Geometry check sheet. Reference: the model listing, model coordinates, mm. Face numbers are marked on the shaded views. A direction names the side the tool comes from. Give positions to 0.01 mm unless a question says otherwise; leave off trailing zeros. Loops run counter-clockwise (first coordinate to the right, second up) from the corner with the lowest first, then second, coordinate; pieces in that order, holes last. Notation, with made-up numbers: (12, 52) -> (71, 52) arc R31 ccw to (71, 76) -> close; hole circle Ø7 at (32, 79). An arc over 180 degrees is marked (long way). One line per item, written item: value. Start each with the question number.
(1) Sectioned sample at B-B, the plane x = -14. Record the cut outline in (y, z) (3 decimals), then the cut area to 3 significant figures.
(2) Scan lines: line 1 along Z through (x, y) = (-53.5, 7) (3 decimals); line 2 along Z through (x, y) = (-17, -2) (3 decimals); line 3 along X through (y, z) = (-17.5, -106). Record each from-to range of solid material in increasing order. Write a range as from..to.
(3) Tool access check on the marked faces 1, 2, 3, 4 and 5. Record the directions out of +Z, -Z, +X, -X, +Y, -Y that give a thin tool (end or side, any length) a straight path to the whole face; none if there is none.
(4) Sectioned sample at C-C, the plane z = -66.5. Record the cut outline in (x, y), then the cut area to 3 significant figures.
(5) Gauge pin test, flat ends, axial feed: pin 1 Ø11.5 at (x, y) = (-24.5, -7.5) entering from -Z; pin 2 Ø10 at (x, z) = (-1.5, -98.5) entering from +Y; pin 3 Ø19 at (y, z) = (8, -49) entering from +X; pin 4 Ø5 at (y, z) = (-9, -111.5) entering from +X. Record the tip position at first contact, or that the pin passes through.
(6) Sectioned sample at D-D, the plane y = -9. State how many separate pieces and enclosed holes the cut face has, then the cut area to 3 significant figures.
(7) Sectioned sample at A-A, the plane x = -39.5. Record the cut outline in (y, z) (3 decimals).
(8) Draft check along X on the marked faces 6, 7, 8 and 9. Enter one of: pulls with the +X half, pulls with the -X half, needs draft (parallel to the pull), parting line crosses it, or undercut.
from build123d import *

# Parameters (mm, degrees)
F1_DEPTH     = 19.05
F6_T1_DEPTH  = 38.1
F6_T3_DEPTH  = 19.05
F6_T5_DEPTH  = 19.05
F6_T10_ANGLE = 45.2137620144
F6_T16_ANGLE = 107.7622686142
F6_T22_ANGLE = 107.7622686142
F6_T25_DEPTH = 69.8548284901
F7_R         = 1.8415
F8_DEPTH     = 38.1010001


# Not quite as in the source:
# - a fillet or chamfer that OpenCascade refuses, or shapes differently, is made with other operations: its cross-section is extruded or revolved along the edge and cut away or added


with BuildPart() as f1:
    # F0 (on Front) → F1 (new body, symmetric)
    with BuildSketch(Plane.XZ):
        Polygon((-63.5, 0), (0, 0), (0, -16.2306), (-63.5, -16.2306), (-63.5, -124.1806), (-25.4, -124.1806), (-25.4, -101.9556), (-31.75, -101.9556), (-31.75, -111.4806), (-50.8, -111.4806), (-50.8, -89.2556), (12.7, -89.2556), (12.7, -70.2056), (6.35, -70.2056), (6.35, -76.5556), (-50.8, -76.5556), (-50.8, -25.7556), (12.7, -25.7556), (12.7, 9.525), (-63.5, 9.525), align=None)
    extrude(amount=F1_DEPTH, both=True)

    # F2 (on Front) → F3 (revolve, cut)
    with BuildSketch(Plane.XZ):
        Polygon((-50.8, -57.5056), (-50.8, -76.5556), (6.35, -76.5556), (6.35, -70.2056), (12.7, -70.2056), (12.7, -57.5056), align=None)
    revolve(axis=Axis((-20.4399991781, 0, -165.4556), (1, 0, 0)), mode=Mode.SUBTRACT)

    # F4 (on Front) → F5 (revolve, cut)
    with BuildSketch(Plane.XZ):
        Polygon((-50.8, -89.2556), (-50.8, -111.4806), (-31.75, -111.4806), (-31.75, -101.9556), (-25.4, -101.9556), (-25.4, -89.2556), align=None)
    revolve(axis=Axis((-41.275, 0, -149.5806), (1, 0, 0)), mode=Mode.SUBTRACT)

    # F6: fillet of radius 6.35 on 13 edges, made by hand

    # F6_s2 → F6_t1 (join)
    with BuildSketch(Plane.XZ.offset(-19.05)):
        with BuildLine():
            ThreePointArc((-44.4490343146, -25.7552), (-48.9401280605, -27.6154719395), (-50.8004, -32.1065656854))
            Line((-50.8004, -32.1065656854), (-51.4355365685, -32.1065656854))
            ThreePointArc((-51.4355365685, -32.1065656854), (-51.4351365685, -28.9310828427), (-51.4351365685, -25.7556))
            Line((-51.4351365685, -25.7556), (-50.8, -25.1204634315))
            ThreePointArc((-50.8, -25.1204634315), (-47.6245171573, -25.1204634315), (-44.4490343146, -25.1200634315))
            Line((-44.4490343146, -25.1200634315), (-44.4490343146, -25.7552))
        make_face()
    extrude(amount=F6_T1_DEPTH)

    # F6_s4 → F6_t3 (join)
    with BuildSketch(Plane.XZ.offset(-19.05)):
        with BuildLine():
            ThreePointArc((-44.4490343146, -89.2552), (-48.9401280605, -91.1154719395), (-50.8004, -95.6065656854))
            Line((-50.8004, -95.6065656854), (-51.4355365685, -95.6065656854))
            ThreePointArc((-51.4355365685, -95.6065656854), (-51.4351365685, -92.4310828427), (-51.4351365685, -89.2556))
            Line((-51.4351365685, -89.2556), (-50.8, -88.6204634315))
            ThreePointArc((-50.8, -88.6204634315), (-47.6245171573, -88.6204634315), (-44.4490343146, -88.6200634315))
            Line((-44.4490343146, -88.6200634315), (-44.4490343146, -89.2552))
        make_face()
    extrude(amount=F6_T3_DEPTH)

    # F6_s6 → F6_t5 (join)
    with BuildSketch(Plane.XZ):
        with BuildLine():
            ThreePointArc((-44.4490343146, -89.2552), (-48.9401280605, -91.1154719395), (-50.8004, -95.6065656854))
            Line((-50.8004, -95.6065656854), (-51.4355365685, -95.6065656854))
            ThreePointArc((-51.4355365685, -95.6065656854), (-51.4351365685, -92.4310828427), (-51.4351365685, -89.2556))
            Line((-51.4351365685, -89.2556), (-50.8, -88.6204634315))
            ThreePointArc((-50.8, -88.6204634315), (-47.6245171573, -88.6204634315), (-44.4490343146, -88.6200634315))
            Line((-44.4490343146, -88.6200634315), (-44.4490343146, -89.2552))
        make_face()
    extrude(amount=F6_T5_DEPTH)


with BuildPart() as f6_tool8:
    # F6_s9 → F6_t10 (revolve)
    with BuildSketch(Plane(origin=(0, -58.7152257849, -24.4490632784), x_dir=(1, 0, 0), z_dir=(0, -0.923164058, -0.384406194))):
        with BuildLine():
            ThreePointArc((-50.8004, -57.4916974353), (-48.9401280605, -61.9827911812), (-44.4490343146, -63.8430631207))
            Line((-44.4490343146, -63.8430631207), (-44.4490343146, -64.4781996892))
            ThreePointArc((-44.4490343146, -64.4781996892), (-47.6245171573, -64.4777996892), (-50.8, -64.4777996892))
            Line((-50.8, -64.4777996892), (-51.4351365685, -63.8426631207))
            ThreePointArc((-51.4351365685, -63.8426631207), (-51.4351365685, -60.667180278), (-51.4355365685, -57.4916974353))
            Line((-51.4355365685, -57.4916974353), (-50.8004, -57.4916974353))
        make_face()
    revolve(axis=Axis((-50.8, 0, -165.4556), (-1, 0, 0)), revolution_arc=F6_T10_ANGLE)

    split(bisect_by=Plane.XZ.offset(19.05), keep=Keep.BOTTOM)

    split(bisect_by=Plane.XZ.offset(-19.05), keep=Keep.TOP)


with BuildPart() as f1_1:
    add(f1.part)

    # F6_t7: union F6_tool8
    add(f6_tool8.part)


with BuildPart() as f6_tool14:
    # F6_s15 → F6_t16 (revolve)
    with BuildSketch(Plane(origin=(0, -71.2250836382, -97.6064441708), x_dir=(1, 0, 0), z_dir=(0, -0.589462371, -0.8077958363))):
        with BuildLine():
            ThreePointArc((-50.8004, -43.7211694448), (-48.9401280605, -48.2122631908), (-44.4490343146, -50.0725351302))
            Line((-44.4490343146, -50.0725351302), (-44.4490343146, -50.7076716988))
            ThreePointArc((-44.4490343146, -50.7076716988), (-47.6245171573, -50.7072716988), (-50.8, -50.7072716988))
            Line((-50.8, -50.7072716988), (-51.4351365685, -50.0721351302))
            ThreePointArc((-51.4351365685, -50.0721351302), (-51.4351365685, -46.8966522875), (-51.4355365685, -43.7211694448))
            Line((-51.4355365685, -43.7211694448), (-50.8004, -43.7211694448))
        make_face()
    revolve(axis=Axis((-50.8, 0, -149.5806), (-1, 0, 0)), revolution_arc=F6_T16_ANGLE)

    split(bisect_by=Plane.XZ.offset(19.05), keep=Keep.BOTTOM)

    split(bisect_by=Plane.XZ.offset(-19.05), keep=Keep.TOP)


with BuildPart() as f1_2:
    add(f1_1.part)

    # F6_t13: union F6_tool14
    add(f6_tool14.part)


with BuildPart() as f6_tool20:
    # F6_s21 → F6_t22 (revolve)
    with BuildSketch(Plane(origin=(0, -71.2250836382, -97.6064441708), x_dir=(1, 0, 0), z_dir=(0, -0.589462371, -0.8077958363))):
        with BuildLine():
            ThreePointArc((-38.1009656854, -50.0725351302), (-33.6098719395, -48.2122631908), (-31.7496, -43.7211694448))
            Line((-31.7496, -43.7211694448), (-31.1144634315, -43.7211694448))
            ThreePointArc((-31.1144634315, -43.7211694448), (-31.1148634315, -46.8966522875), (-31.1148634315, -50.0721351302))
            Line((-31.1148634315, -50.0721351302), (-31.75, -50.7072716988))
            ThreePointArc((-31.75, -50.7072716988), (-34.9254828427, -50.7072716988), (-38.1009656854, -50.7076716988))
            Line((-38.1009656854, -50.7076716988), (-38.1009656854, -50.0725351302))
        make_face()
    revolve(axis=Axis((-31.75, 0, -149.5806), (-1, 0, 0)), revolution_arc=F6_T22_ANGLE)

    split(bisect_by=Plane.XZ.offset(19.05), keep=Keep.BOTTOM)

    split(bisect_by=Plane.XZ.offset(-19.05), keep=Keep.TOP)


with BuildPart() as f1_3:
    add(f1_2.part)

    # F6_t19: union F6_tool20
    add(f6_tool20.part)

    # F6_s26 → F6_t25 (cut)
    with BuildSketch(Plane.XZ.offset(-34.9274142451)):
        with BuildLine():
            ThreePointArc((6.3490343146, 9.5254), (10.8401280605, 7.6651280605), (12.7004, 3.1740343146))
            Line((12.7004, 3.1740343146), (13.3355365685, 3.1740343146))
            ThreePointArc((13.3355365685, 3.1740343146), (13.3351365685, 6.3495171573), (13.3351365685, 9.525))
            Line((13.3351365685, 9.525), (12.7, 10.1601365685))
            ThreePointArc((12.7, 10.1601365685), (9.5245171573, 10.1601365685), (6.3490343146, 10.1605365685))
            Line((6.3490343146, 10.1605365685), (6.3490343146, 9.5254))
        make_face()
        with BuildLine():
            ThreePointArc((-57.1490343146, 9.5254), (-61.6401280605, 7.6651280605), (-63.5004, 3.1740343146))
            Line((-63.5004, 3.1740343146), (-64.1355365685, 3.1740343146))
            ThreePointArc((-64.1355365685, 3.1740343146), (-64.1351365685, 6.3495171573), (-64.1351365685, 9.525))
            Line((-64.1351365685, 9.525), (-63.5, 10.1601365685))
            ThreePointArc((-63.5, 10.1601365685), (-60.3245171573, 10.1601365685), (-57.1490343146, 10.1605365685))
            Line((-57.1490343146, 10.1605365685), (-57.1490343146, 9.5254))
        make_face()
        with BuildLine():
            ThreePointArc((-63.5004, -22.5815656854), (-61.6401280605, -18.0904719395), (-57.1490343146, -16.2302))
            Line((-57.1490343146, -16.2302), (-57.1490343146, -15.5950634315))
            ThreePointArc((-57.1490343146, -15.5950634315), (-60.3245171573, -15.5954634315), (-63.5, -15.5954634315))
            Line((-63.5, -15.5954634315), (-64.1351365685, -16.2306))
            ThreePointArc((-64.1351365685, -16.2306), (-64.1351365685, -19.4060828427), (-64.1355365685, -22.5815656854))
            Line((-64.1355365685, -22.5815656854), (-63.5004, -22.5815656854))
        make_face()
        with BuildLine():
            ThreePointArc((12.7004, -19.4046343146), (10.8401280605, -23.8957280605), (6.3490343146, -25.756))
            Line((6.3490343146, -25.756), (6.3490343146, -26.3911365685))
            ThreePointArc((6.3490343146, -26.3911365685), (9.5245171573, -26.3907365685), (12.7, -26.3907365685))
            Line((12.7, -26.3907365685), (13.3351365685, -25.7556))
            ThreePointArc((13.3351365685, -25.7556), (13.3351365685, -22.5801171573), (13.3355365685, -19.4046343146))
            Line((13.3355365685, -19.4046343146), (12.7004, -19.4046343146))
        make_face()
        with BuildLine():
            ThreePointArc((-57.1490343146, -124.181), (-61.6401280605, -122.3207280605), (-63.5004, -117.8296343146))
            Line((-63.5004, -117.8296343146), (-64.1355365685, -117.8296343146))
            ThreePointArc((-64.1355365685, -117.8296343146), (-64.1351365685, -121.0051171573), (-64.1351365685, -124.1806))
            Line((-64.1351365685, -124.1806), (-63.5, -124.8157365685))
            ThreePointArc((-63.5, -124.8157365685), (-60.3245171573, -124.8157365685), (-57.1490343146, -124.8161365685))
            Line((-57.1490343146, -124.8161365685), (-57.1490343146, -124.181))
        make_face()
        with BuildLine():
            ThreePointArc((-25.3996, -117.8296343146), (-27.2598719395, -122.3207280605), (-31.7509656854, -124.181))
            Line((-31.7509656854, -124.181), (-31.7509656854, -124.8161365685))
            ThreePointArc((-31.7509656854, -124.8161365685), (-28.5754828427, -124.8157365685), (-25.4, -124.8157365685))
            Line((-25.4, -124.8157365685), (-24.7648634315, -124.1806))
            ThreePointArc((-24.7648634315, -124.1806), (-24.7648634315, -121.0051171573), (-24.7644634315, -117.8296343146))
            Line((-24.7644634315, -117.8296343146), (-25.3996, -117.8296343146))
        make_face()
        with BuildLine():
            ThreePointArc((12.7004, -82.9046343146), (10.8401280605, -87.3957280605), (6.3490343146, -89.256))
            Line((6.3490343146, -89.256), (6.3490343146, -89.8911365685))
            ThreePointArc((6.3490343146, -89.8911365685), (9.5245171573, -89.8907365685), (12.7, -89.8907365685))
            Line((12.7, -89.8907365685), (13.3351365685, -89.2556))
            ThreePointArc((13.3351365685, -89.2556), (13.3351365685, -86.0801171573), (13.3355365685, -82.9046343146))
            Line((13.3355365685, -82.9046343146), (12.7004, -82.9046343146))
        make_face()
    extrude(amount=F6_T25_DEPTH, mode=Mode.SUBTRACT)

    # F7 (on face) → F8 (cut, through all)
    with BuildSketch(Plane.XZ.offset(19.05)):
        with Locations((-57.9040207225, -100.6856)):
            Circle(F7_R)
        with Locations((-57.9040207225, -113.3856)):
            Circle(F7_R)
    extrude(amount=-F8_DEPTH, mode=Mode.SUBTRACT)


solid = f1_3.part
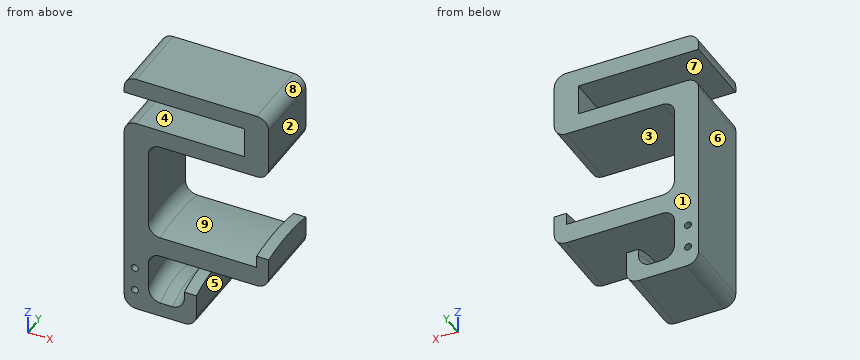
Calculated:
1. outline: (-19.05, -89.256) -> (19.05, -89.256) -> (19.05, -78.621) arc R88.9 ccw to (-19.05, -78.621) -> close; (-19.05, -25.756) -> (19.05, -25.756) -> (19.05, -16.231) -> (-19.05, -16.231) -> close; (-19.05, 0) -> (19.05, 0) -> (19.05, 9.525) -> (-19.05, 9.525) -> close
1. area: 1,180 mm2
2. line 1: z = -124.181..-16.231, 0..9.525
2. line 2: z = -89.256..-76.578, -25.756..-16.231, 0..9.525
2. line 3: x = -63.5..-50.8, -31.75..-25.4
3. face 1: +Z, -Z, +X, -X, +Y
3. face 2: +Z, -Z, +X, +Y, -Y
3. face 3: +X, +Y, -Y
3. face 4: -X, +Y, -Y
3. face 5: -Z, +X, +Y, -Y
4. outline: (-63.5, -19.05) -> (-50.8, -19.05) -> (-50.8, 19.05) -> (-63.5, 19.05) -> close
4. area: 484 mm2
5. pin 1: stops at z = -124
5. pin 2: passes through
5. pin 3: stops at x = -50.8
5. pin 4: stops at x = -25.4
6. separate pieces: 1
6. enclosed holes: 2
6. area: 4,040 mm2
7. outline: (-19.05, -124.181) -> (19.05, -124.181) -> (19.05, -116.585) arc R38.1 ccw to (-19.05, -116.585) -> close; (-19.05, -89.256) -> (19.05, -89.256) -> (19.05, -78.621) arc R88.9 ccw to (-19.05, -78.621) -> close; (-19.05, -25.756) -> (19.05, -25.756) -> (19.05, -16.231) -> (-19.05, -16.231) -> close; (-19.05, 0) -> (19.05, 0) -> (19.05, 9.525) -> (-19.05, 9.525) -> close
8. face 6: pulls with the -X half
8. face 7: needs draft
8. face 8: pulls with the +X half
8. face 9: undercut
